The listing builds one solid part. Answer for the finished solid, in the listing's coordinates (mm). A direction names the side the tool comes from. Give positions to 0.01 mm unless a question says otherwise; leave off trailing zeros. Order: outer loops, then holes, each group sorted by start corner. A loop starts at its lowest first (then second) coordinate and runs counter-clockwise, first axis right, second up.
```python
from build123d import *

# Parameters (mm, degrees)
SKETCH1_W           = 76.2
SKETCH1_H           = 31.75
BOSS_EXTRUDE1_DEPTH = 3.175
SKETCH2_R           = 0.508
SKETCH2_W           = 3.175
SKETCH2_H           = 16.51
CUT_EXTRUDE1_DEPTH  = 3.175


with BuildPart() as part:
    # Sketch1 → Boss-Extrude1 (new body)
    with BuildSketch(Plane(origin=(0, 0, 0), x_dir=(1, 0, 0), z_dir=(0, 1, 0))):
        Rectangle(SKETCH1_W, SKETCH1_H)
    extrude(amount=BOSS_EXTRUDE1_DEPTH)

    # Sketch2 → Cut-Extrude1 (cut)
    with BuildSketch(Plane(origin=(0, 3.175, 0), x_dir=(1, 0, 0), z_dir=(0, 1, 0))):
        with Locations(Location((30.737005641, 9.525, 0), (0, 0, 270))):
            Circle(SKETCH2_R)
        with Locations(Location((30.737005641, -9.525, 0), (0, 0, 270))):
            Circle(SKETCH2_R)
        with Locations(Location((11.687005641, 9.525, 0), (0, 0, 270))):
            Circle(SKETCH2_R)
        with Locations(Location((11.687005641, -9.525, 0), (0, 0, 270))):
            Circle(SKETCH2_R)
        with Locations((-36.5125, 0)):
            Rectangle(SKETCH2_W, SKETCH2_H)
    extrude(amount=-CUT_EXTRUDE1_DEPTH, mode=Mode.SUBTRACT)


solid = part.part
```
1) For a pull along Z with two mould halves and no side action, classify faces 3 (the flat face through (-1, 0, 0)), 4 (the flat face through (-1, 2, 15.875)), 5 (the flat face through (-34.925, 2, 0)), 6 (the flat face through (-37, 2, 8.255)) as +Z half, -Z half, draft (parallel to the pull), parting line (faces both ways), or undercut.
Geometry says:
face 3: draft
face 4: +Z half
face 5: undercut
face 6: undercut
2) Find section A-A (y = 1.45). Write down the section's boundary in (x, z) (3 decimals), then the cut area to 3 significant figures.
Geometry says:
outline: (-38.1, -15.875) - (38.1, -15.875) - (38.1, 15.875) - (-38.1, 15.875) - (-38.1, 8.255) - (-34.925, 8.255) - (-34.925, -8.255) - (-38.1, -8.255) - close; hole circle Ø1.016 at (11.687, -9.525); hole circle Ø1.016 at (11.687, 9.525); hole circle Ø1.016 at (30.737, -9.525); hole circle Ø1.016 at (30.737, 9.525)
area: 2,360 mm2
3) Find section B-B (z = -5). Write down the section's boundary in (x, y) (3 decimals), then the cut area to 3 significant figures.
Geometry says:
outline: (-34.925, 0) - (38.1, 0) - (38.1, 3.175) - (-34.925, 3.175) - close
area: 232 mm2
4) Given P1, Ø1.2, axis at x = 11.69, z = -9.52, coming from the +Y side (3 decimals), flat-ended and moving along its own axis, determine where the tip first touches the part or whether it passes through.
Geometry says:
P1: stops at y = 3.175
5) A tool of negligible diameter and unlimited length cuts with its end or side. For faces 1 (the flat face through (-37, 2, -8.255)), 2 (the flat face through (-1, 3.175, 0)), from which of +Z, -Z, +X, -X, +Y, -Y can it reach the whole face along a straight path? Write none if from no direction.
Geometry says:
face 1: -X, +Y, -Y
face 2: +Z, -Z, +X, -X, +Y
6) Straight lines are drawn through the part: probe 1 along X at (y, z) = (1.75, -3) (3 decimals); probe 2 along Z at (x, y) = (12, 1.05) (3 decimals). For each, find the intervals that lie inside material, in ascending order.
Geometry says:
probe 1: x = -34.925 to 38.1
probe 2: z = -15.875 to -9.925, -9.125 to 9.125, 9.925 to 15.875
